Could you check a few things on this model? Use its own coordinates, in mm. A direction names the side the tool comes from. Give positions to 0.01 mm unless a question says otherwise; leave off trailing zeros. Write each loop counter-clockwise with the first axis right and the second up, starting at its lowest first coordinate (ties: lowest second). Pieces come first, ordered by that corner, then holes. Notation, with made-up numbers: (16.25, -19) - (50.25, -19) arc R12 ccw to (50.25, 1) - close; hole circle Ø11 at (84.5, 11.25). An arc over 180 degrees is marked (long way). Use one line per item in the form item = value.
```python
from build123d import *

# Parameters (mm, degrees)
F0_R     = 7.5
F1_DEPTH = 4


with BuildPart() as f1:
    # F0 (on Top) → F1 (new body)
    with BuildSketch(Plane.XY):
        with BuildLine():
            ThreePointArc((10.5023390129, 4.6851761182), (10.0305689983, 5.3963431452), (9.6971069971, 6.1819184634))
            ThreePointArc((9.6971069971, 6.1819184634), (8.1317279836, 8.1317279836), (6.1819184634, 9.6971069971))
            ThreePointArc((6.1819184634, 9.6971069971), (5.3963431452, 10.0305689983), (4.6851761182, 10.5023390129))
            ThreePointArc((4.6851761182, 10.5023390129), (0, 11.5), (-4.6851761182, 10.5023390129))
            ThreePointArc((-4.6851761182, 10.5023390129), (-5.3963431452, 10.0305689983), (-6.1819184634, 9.6971069971))
            ThreePointArc((-6.1819184634, 9.6971069971), (-8.1317279836, 8.1317279836), (-9.6971069971, 6.1819184634))
            ThreePointArc((-9.6971069971, 6.1819184634), (-10.0305689983, 5.3963431452), (-10.5023390129, 4.6851761182))
            ThreePointArc((-10.5023390129, 4.6851761182), (-11.5, 0), (-10.5023390129, -4.6851761182))
            ThreePointArc((-10.5023390129, -4.6851761182), (-10.0305689983, -5.3963431452), (-9.6971069971, -6.1819184634))
            ThreePointArc((-9.6971069971, -6.1819184634), (-8.1317279836, -8.1317279836), (-6.1819184634, -9.6971069971))
            ThreePointArc((-6.1819184634, -9.6971069971), (-5.3963431452, -10.0305689983), (-4.6851761182, -10.5023390129))
            ThreePointArc((-4.6851761182, -10.5023390129), (0, -11.5), (4.6851761182, -10.5023390129))
            ThreePointArc((4.6851761182, -10.5023390129), (5.3963431452, -10.0305689983), (6.1819184634, -9.6971069971))
            ThreePointArc((6.1819184634, -9.6971069971), (8.1317279836, -8.1317279836), (9.6971069971, -6.1819184634))
            ThreePointArc((9.6971069971, -6.1819184634), (10.0305689983, -5.3963431452), (10.5023390129, -4.6851761182))
            ThreePointArc((10.5023390129, -4.6851761182), (11.2478197587, -2.3951097419), (11.5, 0))
            ThreePointArc((11.5, 0), (11.2478197587, 2.3951097419), (10.5023390129, 4.6851761182))
        make_face()
        Circle(F0_R, mode=Mode.SUBTRACT)
        with BuildLine():
            ThreePointArc((14.6103055623, 2.982595382), (12.338941223, 3.3093913031), (10.5023390129, 4.6851761182))
            ThreePointArc((10.5023390129, 4.6851761182), (11.2478197587, 2.3951097419), (11.5, 0))
            ThreePointArc((11.5, 0), (11.2478197587, -2.3951097419), (10.5023390129, -4.6851761182))
            ThreePointArc((10.5023390129, -4.6851761182), (12.2847026286, -3.3322754018), (14.4930952607, -2.9714951504))
            ThreePointArc((14.4930952607, -2.9714951504), (15.6148030882, -3.2054073782), (16.6449174053, -3.7072119959))
            ThreePointArc((16.6449174053, -3.7072119959), (15, 0), (16.6449174053, 3.7072119959))
            ThreePointArc((16.6449174053, 3.7072119959), (15.6703838257, 3.2248055408), (14.6103055623, 2.982595382))
        make_face()
        with BuildLine():
            ThreePointArc((-4.6851761182, 10.5023390129), (0, 11.5), (4.6851761182, 10.5023390129))
            ThreePointArc((4.6851761182, 10.5023390129), (3.3322754018, 12.2847026286), (2.9714951504, 14.4930952607))
            ThreePointArc((2.9714951504, 14.4930952607), (3.2054073782, 15.6148030882), (3.7072119959, 16.6449174053))
            ThreePointArc((3.7072119959, 16.6449174053), (0, 15), (-3.7072119959, 16.6449174053))
            ThreePointArc((-3.7072119959, 16.6449174053), (-3.2248055408, 15.6703838257), (-2.982595382, 14.6103055623))
            ThreePointArc((-2.982595382, 14.6103055623), (-3.3093913031, 12.338941223), (-4.6851761182, 10.5023390129))
        make_face()
        with BuildLine():
            Line((14.9337128596, 4.5302571293), (14.6103055623, 2.982595382))
            ThreePointArc((14.6103055623, 2.982595382), (15.6703838257, 3.2248055408), (16.6449174053, 3.7072119959))
            ThreePointArc((16.6449174053, 3.7072119959), (16.936960195, 3.9519346089), (17.2467904427, 4.17370784))
            ThreePointArc((17.2467904427, 4.17370784), (22.3700160562, 4.4026155741), (25, 0))
            ThreePointArc((25, 0), (22.3700160562, -4.4026155741), (17.2467904427, -4.17370784))
            ThreePointArc((17.2467904427, -4.17370784), (16.936960195, -3.9519346089), (16.6449174053, -3.7072119959))
            ThreePointArc((16.6449174053, -3.7072119959), (15.6148030882, -3.2054073782), (14.4930952607, -2.9714951504))
            Line((14.4930952607, -2.9714951504), (18.6098258106, -6.6526619311))
            Line((18.6098258106, -6.6526619311), (25.0662871404, -4.5302571293))
            Line((25.0662871404, -4.5302571293), (26.4564613299, 2.1224048018))
            Line((26.4564613299, 2.1224048018), (21.3901741894, 6.6526619311))
            Line((21.3901741894, 6.6526619311), (14.9337128596, 4.5302571293))
        make_face()
        with BuildLine():
            ThreePointArc((3.7072119959, 16.6449174053), (3.2054073782, 15.6148030882), (2.9714951504, 14.4930952607))
            Line((2.9714951504, 14.4930952607), (6.6526619311, 18.6098258106))
            Line((6.6526619311, 18.6098258106), (4.5302571293, 25.0662871404))
            Line((4.5302571293, 25.0662871404), (-2.1224048018, 26.4564613299))
            Line((-2.1224048018, 26.4564613299), (-6.6526619311, 21.3901741894))
            Line((-6.6526619311, 21.3901741894), (-4.5302571293, 14.9337128596))
            Line((-4.5302571293, 14.9337128596), (-2.982595382, 14.6103055623))
            ThreePointArc((-2.982595382, 14.6103055623), (-3.2248055408, 15.6703838257), (-3.7072119959, 16.6449174053))
            ThreePointArc((-3.7072119959, 16.6449174053), (-3.9519346089, 16.936960195), (-4.17370784, 17.2467904427))
            ThreePointArc((-4.17370784, 17.2467904427), (-1.4372649025, 24.7889737523), (5, 20))
            ThreePointArc((5, 20), (4.7889737523, 18.5627350975), (4.17370784, 17.2467904427))
            ThreePointArc((4.17370784, 17.2467904427), (3.9519346089, 16.936960195), (3.7072119959, 16.6449174053))
        make_face()
        with BuildLine():
            ThreePointArc((-10.5023390129, -4.6851761182), (-11.5, 0), (-10.5023390129, 4.6851761182))
            ThreePointArc((-10.5023390129, 4.6851761182), (-12.2847026286, 3.3322754018), (-14.4930952607, 2.9714951504))
            ThreePointArc((-14.4930952607, 2.9714951504), (-15.6148030882, 3.2054073782), (-16.6449174053, 3.7072119959))
            ThreePointArc((-16.6449174053, 3.7072119959), (-15.4296929549, 2.0278790677), (-15, 0))
            ThreePointArc((-15, 0), (-15.4296929549, -2.0278790677), (-16.6449174053, -3.7072119959))
            ThreePointArc((-16.6449174053, -3.7072119959), (-15.6703838257, -3.2248055408), (-14.6103055623, -2.982595382))
            ThreePointArc((-14.6103055623, -2.982595382), (-12.338941223, -3.3093913031), (-10.5023390129, -4.6851761182))
        make_face()
        with BuildLine():
            ThreePointArc((2.982595382, -14.6103055623), (3.3093913031, -12.338941223), (4.6851761182, -10.5023390129))
            ThreePointArc((4.6851761182, -10.5023390129), (0, -11.5), (-4.6851761182, -10.5023390129))
            ThreePointArc((-4.6851761182, -10.5023390129), (-3.3322754018, -12.2847026286), (-2.9714951504, -14.4930952607))
            ThreePointArc((-2.9714951504, -14.4930952607), (-3.2054073782, -15.6148030882), (-3.7072119959, -16.6449174053))
            ThreePointArc((-3.7072119959, -16.6449174053), (0, -15), (3.7072119959, -16.6449174053))
            ThreePointArc((3.7072119959, -16.6449174053), (3.2248055408, -15.6703838257), (2.982595382, -14.6103055623))
        make_face()
        with BuildLine():
            ThreePointArc((-16.6449174053, 3.7072119959), (-15.6148030882, 3.2054073782), (-14.4930952607, 2.9714951504))
            Line((-14.4930952607, 2.9714951504), (-18.6098258106, 6.6526619311))
            Line((-18.6098258106, 6.6526619311), (-25.0662871404, 4.5302571293))
            Line((-25.0662871404, 4.5302571293), (-26.4564613299, -2.1224048018))
            Line((-26.4564613299, -2.1224048018), (-21.3901741894, -6.6526619311))
            Line((-21.3901741894, -6.6526619311), (-14.9337128596, -4.5302571293))
            Line((-14.9337128596, -4.5302571293), (-14.6103055623, -2.982595382))
            ThreePointArc((-14.6103055623, -2.982595382), (-15.6703838257, -3.2248055408), (-16.6449174053, -3.7072119959))
            ThreePointArc((-16.6449174053, -3.7072119959), (-16.936960195, -3.9519346089), (-17.2467904427, -4.17370784))
            ThreePointArc((-17.2467904427, -4.17370784), (-25, 0), (-17.2467904427, 4.17370784))
            ThreePointArc((-17.2467904427, 4.17370784), (-16.936960195, 3.9519346089), (-16.6449174053, 3.7072119959))
        make_face()
        with BuildLine():
            Line((4.5302571293, -14.9337128596), (2.982595382, -14.6103055623))
            ThreePointArc((2.982595382, -14.6103055623), (3.2248055408, -15.6703838257), (3.7072119959, -16.6449174053))
            ThreePointArc((3.7072119959, -16.6449174053), (3.9519346089, -16.936960195), (4.17370784, -17.2467904427))
            ThreePointArc((4.17370784, -17.2467904427), (4.7889737523, -18.5627350975), (5, -20))
            ThreePointArc((5, -20), (-1.4372649025, -24.7889737523), (-4.17370784, -17.2467904427))
            ThreePointArc((-4.17370784, -17.2467904427), (-3.9519346089, -16.936960195), (-3.7072119959, -16.6449174053))
            ThreePointArc((-3.7072119959, -16.6449174053), (-3.2054073782, -15.6148030882), (-2.9714951504, -14.4930952607))
            Line((-2.9714951504, -14.4930952607), (-6.6526619311, -18.6098258106))
            Line((-6.6526619311, -18.6098258106), (-4.5302571293, -25.0662871404))
            Line((-4.5302571293, -25.0662871404), (2.1224048018, -26.4564613299))
            Line((2.1224048018, -26.4564613299), (6.6526619311, -21.3901741894))
            Line((6.6526619311, -21.3901741894), (4.5302571293, -14.9337128596))
        make_face()
    extrude(amount=F1_DEPTH)


solid = f1.part
```
1. Which directions (+Z, -Z, +X, -X, +Y, -Y) give clear straight access to the entire face, cutting with the end or side of a thin tool? Please do faces 4 (the face through (4.356, -23.959, 1.972)), 5 (the face through (16.523, -4.786, 1.972)), 6 (the face through (18.207, 5.606, 1.972)), 7 (the face through (3.767, -14.774, 1.972)), 8 (the face through (0, -8, 4)).
Response values:
face_4 = +Z, -Z, +X, -Y
face_5 = +Z, -Z, -Y
face_6 = +Z, -Z, +Y
face_7 = +Z, -Z, +X
face_8 = +Z, +X, -X, +Y, -Y
2. Imagine slicing it at C-C, the plane x = 0. List the corners of the cut face in (y, z) for me.
Response values:
outline = (-26.01, 0) - (-25, 0) - (-25, 4) - (-26.01, 4) - close; (-15, 0) - (-7.5, 0) - (-7.5, 4) - (-15, 4) - close; (7.5, 0) - (15, 0) - (15, 4) - (7.5, 4) - close; (25, 0) - (26.01, 0) - (26.01, 4) - (25, 4) - close
3. Imagine slicing it at D-D, the plane z = 2.9. State how many separate pieces and enclosed holes the cut face has, and give its area (3 significant figures).
Response values:
separate_pieces = 1
enclosed_holes = 5
area = 478 mm²
4. For pin 1 (9 mm diameter, centred on x = 0, y = 20, fed in from +Z); pin 2 (1.5 mm diameter, centred on x = -7.5, z = 2.5, fed in from -Y), each with a flat end and sliding along its axis, tell me the tip position at first contact or that it passes through.
Response values:
pin_1 = through
pin_2 = -9.31
5. If we mould it in two halves opening along Y, with no side actions, what happens to faces 1 (the face through (-23.959, -4.356, 1.972)), 2 (the face through (-4.786, -16.523, 1.972)), 3 (the face through (-4.356, 23.959, 1.972))? For each: pulls with the +Y half, pulls with the -Y half, needs draft (parallel to the pull), parting line crosses it, or undercut.
Response values:
face_1 = pulls with the -Y half
face_2 = undercut
face_3 = pulls with the +Y half
6. If I drill on line 1 (X direction, y = 20, z = 1.5); line 2 (Y direction, x = 0.5, z = 2.25); line 3 (X direction, y = 2.5, z = 3.5), over which ranges is the centre line in solid material (lowest first)? Write a range as from..to.
Response values:
line_1 = -6.2..-5, 5..6.2
line_2 = -26.12..-24.97, -15.03..-7.48, 7.48..15.03, 24.97..25.91
line_3 = -25.49..-24.33, -15.67..-7.07, 7.07..15.67, 24.33..26.03
7. Imagine slicing it at B-B, the plane y = 16. List the corners of the cut face in (x, z) for me, and give its area (3 significant figures).
Response values:
outline = (-4.88, 0) - (-3, 0) - (-3, 4) - (-4.88, 4) - close; (3, 0) - (4.32, 0) - (4.32, 4) - (3, 4) - close
area = 12.8 mm²
8. Imagine slicing it at A-A, the plane x = -20. List the corners of the cut face in (y, z) for me, and give its area (3 significant figures).
Response values:
outline = (-6.2, 0) - (-5, 0) - (-5, 4) - (-6.2, 4) - close; (5, 0) - (6.2, 0) - (6.2, 4) - (5, 4) - close
area = 9.57 mm²
